```python
from build123d import *

# Parameters (mm, degrees)
CYLINDER217_R             = 0.8
CYLINDER217_DEPTH         = 5
CYLINDER218_R             = 0.8
CYLINDER218_DEPTH         = 5
CYLINDER216_R             = 0.8
CYLINDER216_DEPTH         = 5
CYLINDER215_R             = 1.55
CYLINDER215_DEPTH         = 47
CYLINDER214_R             = 3
CYLINDER214_DEPTH         = 4
BOX140_W                  = 6
BOX140_H                  = 16
BOX140_DEPTH              = 10
BOX143_W                  = 10
BOX143_H                  = 6
BOX143_DEPTH              = 11
BOX142_W                  = 10
BOX142_H                  = 10
BOX142_DEPTH              = 9
CYLINDER213_R             = 12.5
CYLINDER213_DEPTH         = 6
BOX141_W                  = 20
BOX141_H                  = 10
BOX141_DEPTH              = 26
CYLINDER212_R             = 2.75
CYLINDER212_DEPTH         = 30
BOX139_W                  = 10
BOX139_H                  = 10
BOX139_DEPTH              = 10
CYLINDER211_R             = 2
CYLINDER211_DEPTH         = 92
BOX138_W                  = 10
BOX138_H                  = 60
BOX138_DEPTH              = 10
CYLINDER210_R             = 1.6
CYLINDER210_DEPTH         = 10
CYLINDER209_R             = 1.6
CYLINDER209_DEPTH         = 10
CYLINDER208_R             = 1.6
CYLINDER208_DEPTH         = 10
CYLINDER207_R             = 1.6
CYLINDER207_DEPTH         = 10
CYLINDER206_R             = 1.6
CYLINDER206_DEPTH         = 92
BOX133_W                  = 10
BOX133_H                  = 12.5
BOX133_DEPTH              = 12
BOX131_W                  = 2
BOX131_H                  = 16
BOX131_DEPTH              = 26
BOX132_W                  = 4
BOX132_H                  = 16
BOX132_DEPTH              = 14
BOX130_W                  = 12
BOX130_H                  = 16
BOX130_DEPTH              = 12
BOX135_W                  = 8
BOX135_H                  = 2
BOX135_DEPTH              = 6
BOX134_W                  = 8
BOX134_H                  = 2
BOX134_DEPTH              = 6
FILLET057_R               = 2.5
BOX137_W                  = 8
BOX137_H                  = 2
BOX137_DEPTH              = 6
BOX136_W                  = 8
BOX136_H                  = 2
BOX136_DEPTH              = 6
FILLET058_R               = 2.5
BOX129_W                  = 10
BOX129_H                  = 12.5
BOX129_DEPTH              = 12
BOX127_W                  = 2
BOX127_H                  = 16
BOX127_DEPTH              = 26
BOX128_W                  = 4
BOX128_H                  = 16
BOX128_DEPTH              = 14
BOX126_W                  = 12
BOX126_H                  = 16
BOX126_DEPTH              = 12
FILLET056_R               = 3
FILLET055_R               = 4
FILLET055_PLACEMENT_ANGLE = 3


with BuildPart() as cylinder512:
    # Cylinder217 → Cylinder217 (new body)
    with BuildSketch(Plane(origin=(331, 23, -46), x_dir=(0, 0, -1), z_dir=(1, 0, 0))):
        Circle(CYLINDER217_R)
    extrude(amount=CYLINDER217_DEPTH)


with BuildPart() as cylinder513:
    # Cylinder218 → Cylinder218 (new body)
    with BuildSketch(Plane(origin=(331, 8, -29), x_dir=(0, 0, -1), z_dir=(1, 0, 0))):
        Circle(CYLINDER218_R)
    extrude(amount=CYLINDER218_DEPTH)


with BuildPart() as fusion188:
    # Cylinder216 → Cylinder216 (new body)
    with BuildSketch(Plane(origin=(331, 8, -54), x_dir=(0, 0, -1), z_dir=(1, 0, 0))):
        Circle(CYLINDER216_R)
    extrude(amount=CYLINDER216_DEPTH)

    # Fusion188: union Cylinder512, Cylinder513
    add(cylinder512.part)
    add(cylinder513.part)


with BuildPart() as cylinder509:
    # Cylinder215 → Cylinder215 (new body)
    with BuildSketch(Plane(origin=(333.25, 20, -34.25), x_dir=(1, 0, 0), z_dir=(0, -1, 0))):
        Circle(CYLINDER215_R)
    extrude(amount=CYLINDER215_DEPTH)


with BuildPart() as cylinder510:
    # Cylinder214 → Cylinder214 (new body)
    with BuildSketch(Plane(origin=(332, 2, -39), x_dir=(0, 0, -1), z_dir=(1, 0, 0))):
        Circle(CYLINDER214_R)
    extrude(amount=CYLINDER214_DEPTH)


with BuildPart() as cube247:
    # Box140 → Box140 (new body)
    with BuildSketch(Plane(origin=(330, -6, -37), x_dir=(1, 0, 0), z_dir=(0, 0, 1))):
        with Locations((3, 8)):
            Rectangle(BOX140_W, BOX140_H)
    extrude(amount=BOX140_DEPTH)


with BuildPart() as cube246:
    # Box143 → Box143 (new body)
    with BuildSketch(Plane(origin=(328, 12, -40), x_dir=(1, 0, 0), z_dir=(0, 0, 1))):
        with Locations((5, 3)):
            Rectangle(BOX143_W, BOX143_H)
    extrude(amount=BOX143_DEPTH)


with BuildPart() as cube245:
    # Box142 → Box142 (new body)
    with BuildSketch(Plane(origin=(326, 10, -36), x_dir=(1, 0, 0), z_dir=(0, 0, 1))):
        with Locations((5, 5)):
            Rectangle(BOX142_W, BOX142_H)
    extrude(amount=BOX142_DEPTH)


with BuildPart() as cylinder507:
    # Cylinder213 → Cylinder213 (new body)
    with BuildSketch(Plane(origin=(329.25, 18, -49), x_dir=(1, 0, 0), z_dir=(0, -1, 0))):
        Circle(CYLINDER213_R)
    extrude(amount=CYLINDER213_DEPTH)


with BuildPart() as cut151:
    # Box141 → Box141 (new body)
    with BuildSketch(Plane(origin=(316, 10, -62), x_dir=(1, 0, 0), z_dir=(0, 0, 1))):
        with Locations((10, 5)):
            Rectangle(BOX141_W, BOX141_H)
    extrude(amount=BOX141_DEPTH)

    # Cut152: cut Cylinder507
    add(cylinder507.part, mode=Mode.SUBTRACT)

    # Fusion187: union Cube245
    add(cube245.part)

    # Cut151: cut Cube246
    add(cube246.part, mode=Mode.SUBTRACT)


with BuildPart() as cut149:
    # Cylinder212 → Cylinder212 (new body)
    with BuildSketch(Plane(origin=(333.25, 10, -34.25), x_dir=(1, 0, 0), z_dir=(0, -1, 0))):
        Circle(CYLINDER212_R)
    extrude(amount=CYLINDER212_DEPTH)

    # Fusion186: union Cube247, Cut151
    add(cube247.part)
    add(cut151.part)

    # Cut150: cut Cylinder510
    add(cylinder510.part, mode=Mode.SUBTRACT)

    # Cut149: cut Cylinder509
    add(cylinder509.part, mode=Mode.SUBTRACT)


with BuildPart() as cube238:
    # Box139 → Box139 (new body)
    with BuildSketch(Plane(origin=(326, 10, -54), x_dir=(1, 0, 0), z_dir=(0, 0, 1))):
        with Locations((5, 5)):
            Rectangle(BOX139_W, BOX139_H)
    extrude(amount=BOX139_DEPTH)


with BuildPart() as cylinder499:
    # Cylinder211 → Cylinder211 (new body)
    with BuildSketch(Plane(origin=(329.25, 86, -49), x_dir=(1, 0, 0), z_dir=(0, -1, 0))):
        Circle(CYLINDER211_R)
    extrude(amount=CYLINDER211_DEPTH)


with BuildPart() as cut148:
    # Box138 → Box138 (new body)
    with BuildSketch(Plane(origin=(326, 10, -54), x_dir=(1, 0, 0), z_dir=(0, 0, 1))):
        with Locations((5, 30)):
            Rectangle(BOX138_W, BOX138_H)
    extrude(amount=BOX138_DEPTH)

    # Cut148: cut Cylinder499
    add(cylinder499.part, mode=Mode.SUBTRACT)


with BuildPart() as cylinder503:
    # Cylinder210 → Cylinder210 (new body)
    with BuildSketch(Plane(origin=(323, 0, -39), x_dir=(0, 0, -1), z_dir=(1, 0, 0))):
        Circle(CYLINDER210_R)
    extrude(amount=CYLINDER210_DEPTH)


with BuildPart() as fusion185:
    # Cylinder209 → Cylinder209 (new body)
    with BuildSketch(Plane(origin=(323, 0, -59), x_dir=(0, 0, -1), z_dir=(1, 0, 0))):
        Circle(CYLINDER209_R)
    extrude(amount=CYLINDER209_DEPTH)

    # Fusion185: union Cylinder503
    add(cylinder503.part)


with BuildPart() as fusion185_1:
    # Fusion185 placement: moved
    add(fusion185.part.moved(Location((3, 78, 0))))


with BuildPart() as cylinder500:
    # Cylinder208 → Cylinder208 (new body)
    with BuildSketch(Plane(origin=(323, 0, -39), x_dir=(0, 0, -1), z_dir=(1, 0, 0))):
        Circle(CYLINDER208_R)
    extrude(amount=CYLINDER208_DEPTH)


with BuildPart() as fusion183:
    # Cylinder207 → Cylinder207 (new body)
    with BuildSketch(Plane(origin=(323, 0, -59), x_dir=(0, 0, -1), z_dir=(1, 0, 0))):
        Circle(CYLINDER207_R)
    extrude(amount=CYLINDER207_DEPTH)

    # Fusion184: union Cylinder500
    add(cylinder500.part)


with BuildPart() as fusion183_1:
    # Fusion184 placement: moved
    add(fusion183.part.moved(Location((3, 2, 0))))

    # Fusion183: union Fusion185
    add(fusion185_1.part)


with BuildPart() as cylinder498:
    # Cylinder206 → Cylinder206 (new body)
    with BuildSketch(Plane(origin=(329.25, 86, -49), x_dir=(1, 0, 0), z_dir=(0, -1, 0))):
        Circle(CYLINDER206_R)
    extrude(amount=CYLINDER206_DEPTH)


with BuildPart() as cube227:
    # Box133 → Box133 (new body)
    with BuildSketch(Plane(origin=(324, -4.25, -55), x_dir=(1, 0, 0), z_dir=(0, 0, 1))):
        with Locations((5, 6.25)):
            Rectangle(BOX133_W, BOX133_H)
    extrude(amount=BOX133_DEPTH)


with BuildPart() as cube225:
    # Box131 → Box131 (new body)
    with BuildSketch(Plane(origin=(330, -6, -62), x_dir=(1, 0, 0), z_dir=(0, 0, 1))):
        with Locations((1, 8)):
            Rectangle(BOX131_W, BOX131_H)
    extrude(amount=BOX131_DEPTH)


with BuildPart() as cube226:
    # Box132 → Box132 (new body)
    with BuildSketch(Plane(origin=(332, -6, -56), x_dir=(1, 0, 0), z_dir=(0, 0, 1))):
        with Locations((2, 8)):
            Rectangle(BOX132_W, BOX132_H)
    extrude(amount=BOX132_DEPTH)


with BuildPart() as cut147:
    # Box130 → Box130 (new body)
    with BuildSketch(Plane(origin=(324, -6, -55), x_dir=(1, 0, 0), z_dir=(0, 0, 1))):
        with Locations((6, 8)):
            Rectangle(BOX130_W, BOX130_H)
    extrude(amount=BOX130_DEPTH)

    # Fusion180: union Cube225, Cube226
    add(cube225.part)
    add(cube226.part)

    # Cut147: cut Cube227
    add(cube227.part, mode=Mode.SUBTRACT)


with BuildPart() as cut147_1:
    # Cut147 placement: moved
    add(cut147.part.moved(Location((0, 76, 0))))


with BuildPart() as cube234:
    # Box135 → Box135 (new body)
    with BuildSketch(Plane(origin=(328, -4.5, -52), x_dir=(1, 0, 0), z_dir=(0, 0, 1))):
        with Locations((4, 1)):
            Rectangle(BOX135_W, BOX135_H)
    extrude(amount=BOX135_DEPTH)


with BuildPart() as fillet057:
    # Box134 → Box134 (new body)
    with BuildSketch(Plane(origin=(328, 6.25, -52), x_dir=(1, 0, 0), z_dir=(0, 0, 1))):
        with Locations((4, 1)):
            Rectangle(BOX134_W, BOX134_H)
    extrude(amount=BOX134_DEPTH)

    # Fusion181: union Cube234
    add(cube234.part)

    # Fillet057
    fillet057_edges = [fillet057.edges().sort_by_distance(p)[0] for p in [
        (328, 7.25, -46),
        (328, 7.25, -52),
        (328, -3.5, -46),
        (328, -3.5, -52),
    ]]
    fillet(fillet057_edges, radius=FILLET057_R)


with BuildPart() as fillet057_1:
    # Fillet057 placement: moved
    add(fillet057.part.moved(Location((-1.5, 0, 0))))


with BuildPart() as cube235:
    # Box137 → Box137 (new body)
    with BuildSketch(Plane(origin=(328, -4.5, -52), x_dir=(1, 0, 0), z_dir=(0, 0, 1))):
        with Locations((4, 1)):
            Rectangle(BOX137_W, BOX137_H)
    extrude(amount=BOX137_DEPTH)


with BuildPart() as fillet058:
    # Box136 → Box136 (new body)
    with BuildSketch(Plane(origin=(328, 6.25, -52), x_dir=(1, 0, 0), z_dir=(0, 0, 1))):
        with Locations((4, 1)):
            Rectangle(BOX136_W, BOX136_H)
    extrude(amount=BOX136_DEPTH)

    # Fusion182: union Cube235
    add(cube235.part)

    # Fillet058
    fillet058_edges = [fillet058.edges().sort_by_distance(p)[0] for p in [
        (328, 7.25, -46),
        (328, 7.25, -52),
        (328, -3.5, -46),
        (328, -3.5, -52),
    ]]
    fillet(fillet058_edges, radius=FILLET058_R)


with BuildPart() as fillet058_1:
    # Fillet058 placement: moved
    add(fillet058.part.moved(Location((-1.5, 76.25, 0))))


with BuildPart() as cube221:
    # Box129 → Box129 (new body)
    with BuildSketch(Plane(origin=(324, -4.25, -55), x_dir=(1, 0, 0), z_dir=(0, 0, 1))):
        with Locations((5, 6.25)):
            Rectangle(BOX129_W, BOX129_H)
    extrude(amount=BOX129_DEPTH)


with BuildPart() as cube223:
    # Box127 → Box127 (new body)
    with BuildSketch(Plane(origin=(330, -6, -62), x_dir=(1, 0, 0), z_dir=(0, 0, 1))):
        with Locations((1, 8)):
            Rectangle(BOX127_W, BOX127_H)
    extrude(amount=BOX127_DEPTH)


with BuildPart() as cube224:
    # Box128 → Box128 (new body)
    with BuildSketch(Plane(origin=(332, -6, -56), x_dir=(1, 0, 0), z_dir=(0, 0, 1))):
        with Locations((2, 8)):
            Rectangle(BOX128_W, BOX128_H)
    extrude(amount=BOX128_DEPTH)


with BuildPart() as obj1:
    # Box126 → Box126 (new body)
    with BuildSketch(Plane(origin=(324, -6, -55), x_dir=(1, 0, 0), z_dir=(0, 0, 1))):
        with Locations((6, 8)):
            Rectangle(BOX126_W, BOX126_H)
    extrude(amount=BOX126_DEPTH)

    # Fusion179: union Cube223, Cube224
    add(cube223.part)
    add(cube224.part)

    # Cut146: cut Cube221
    add(cube221.part, mode=Mode.SUBTRACT)

    # Fusion178: union Cut147, Fillet057, Fillet058
    add(cut147_1.part)
    add(fillet057_1.part)
    add(fillet058_1.part)

    # Cut145: cut Cylinder498
    add(cylinder498.part, mode=Mode.SUBTRACT)

    # Cut144: cut Fusion183
    add(fusion183_1.part, mode=Mode.SUBTRACT)

    # Fusion177: union Cut148
    add(cut148.part)

    # Cut143: cut Cube238
    add(cube238.part, mode=Mode.SUBTRACT)

    # Fusion176: union Cut149
    add(cut149.part)

    # Cut142: cut Fusion188
    add(fusion188.part, mode=Mode.SUBTRACT)

    # Fillet056
    fillet056_edges = [obj1.edges().sort_by_distance(p)[0] for p in [
        (316, 15, -62),
        (326, 15, -27),
        (316, 15, -36),
    ]]
    fillet(fillet056_edges, radius=FILLET056_R)

    # Fillet055
    fillet055_edges = [obj1.edges().sort_by_distance(p)[0] for p in [
        (331, -6, -62),
        (333, -6, -27),
        (331, 70, -36),
        (331, 70, -62),
        (331, 86, -62),
        (331, 86, -36),
    ]]
    fillet(fillet055_edges, radius=FILLET055_R)


with BuildPart() as obj1_1:
    # Fillet055 placement: moved
    add(obj1.part.moved(Location((-80, -9, 0))).rotate(Axis((-80, -9, 0), (0, -1, 0)), FILLET055_PLACEMENT_ANGLE))


solid = obj1_1.part
```
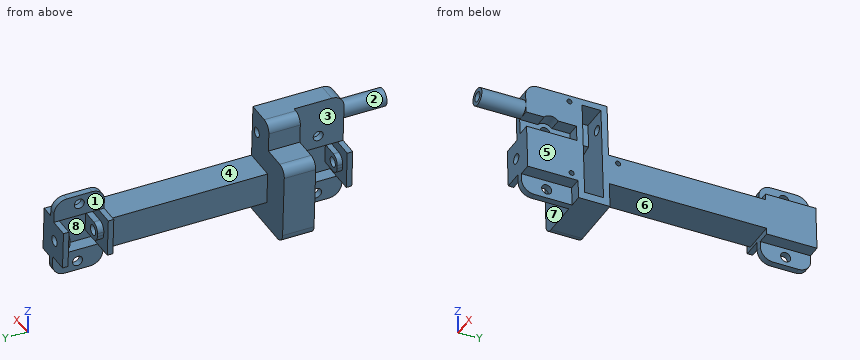
The listing builds one solid part. Answer for the finished solid, in the listing's coordinates (mm). Face numbers are marked on the shaded views. A direction names the side the tool comes from. Coordinates: 2 decimals unless noted, no trailing zeros. Write each loop counter-clockwise with the first axis right and the second up, starting at its lowest first coordinate (ties: lowest second). Pieces come first, ordered by that corner, then holes. Notation, with made-up numbers: (10, 45.5) - (24, 45.5) arc R9 cw to (24, 52.5) - close; hole circle Ø8 at (-2, -28). An arc over 180 degrees is marked (long way). Return JSON: item names as keys, results as strings. Group by question number.
1. A cutting plane is placed at B-B, the plane y = -22. Determine the outline of the cut face in (x, z), plus the area to 3 significant figures.
2. Determine the mould class of the marked faces 5, 6, 7 and 8 for opening direction Y: released by +Y, released by -Y, zero draft, split by the parting line, or undercut.
3. Which of the six approach directions +Z, -Z, +X, -X, +Y, -Y give full straight-line access (tool end or side, diameter ignored) to the marked faces 1, 2, 3 and 4?
4. Given pin 1 (4 mm diameter, centred on x = 254.59, z = -16.76, fed in from +Y); pin 2 (4.5 mm diameter, centred on x = 250.5, z = -32, fed in from -Y); pin 3 (5 mm diameter, centred on x = 253, y = 27.5, fed in from -Z), each flat-ended and moving along its own axis, determine where each tip first touches the part or whether it passes through.
5. Straight lines are drawn through the part: L1, parallel to Y at x = 252.5, z = -30.5; L2, parallel to Y at x = 254.25, z = -30; L3, parallel to Y at x = 249.5, z = -27.5. For each, find the intervals that lie inside material, in ascending order.
6. A cutting plane is placed at A-A, the plane y = 22.5. Determine the outline of the cut face in (x, z).
Ans:
{
 "1": {"outline": "circle Ø5.5 at (254.59, -16.76); hole circle Ø3.1 at (254.59, -16.76)", "area": "16.2 mm²"},
 "2": {"face 5": "zero draft", "face 6": "undercut", "face 7": "released by -Y", "face 8": "undercut"},
 "3": {"face 1": "-X, +Y", "face 2": "-Y", "face 3": "-X, -Y", "face 4": "+Z, -X"},
 "4": {"pin 1": "y = 11", "pin 2": "y = -15", "pin 3": "z = -36.75"},
 "5": {"L1": "-15 to -11.5, -2.75 to 3, 9 to 11, 61 to 64.75, 73.5 to 77", "L2": "-15 to -11.5, -2.75 to 3, 9 to 64.75, 73.5 to 77", "L3": "-15 to -13.25, -0.75 to 3, 9 to 62.75, 75.25 to 77"},
 "6": {"outline": "(247.86, -26.88) - (248.38, -36.86) - (258.37, -36.34) - (257.84, -26.35) - close; hole circle Ø4 at (251.36, -31.7)"}
}
